Could you check a few things on this drawing? It's one solid part, dimensions in mm from its lowest x, y, z. A direction names the side the tool comes from. Give positions to 0.01 mm unless a question says otherwise; leave off trailing zeros. Loops run counter-clockwise (first coordinate to the right, second up) from the corner with the lowest first, then second, coordinate; pieces in that order, holes last. Notation, with made-up numbers: M -10,60.5 L 1,60.5 A20 cw 1,92.5 Z; hole C 6,-6 d4. An arc over 180 degrees is marked long. Answer as CSV lines item,"result". Start each with the question number.
Item 1: Will these pins go through, and if not, where does the flat tip stop? P1, Ø1, axis at x = 4.5, y = 6.5, coming from the +Z side; P2, Ø1, axis at x = 1, y = 4, coming from the +Z side; P3, Ø1.3, axis at x = 5, y = 4, coming from the +Z side; P4, Ø2, axis at x = 2.5, z = 4, coming from the +Y side (1 decimal).
Item 2: I want a section at A-A on z = 3.75. List the corners of the cut face in (x, y) for me (1 decimal).
Item 3: For the marked faces 1, 2 and 3, which set-ups out of +Z, -Z, +X, -X, +Y, -Y let a thin tool reach every point of the face, with its end or its side?
Item 4: I want a section at D-D on x = 1.5. List the corners of the cut face in (y, z) for me (1 decimal).
Item 5: I want a section at C-C on z = 1. List the corners of the cut face in (x, y) for me (1 decimal), plus the area to 3 significant figures.
Item 6: If I drill on line 1 along X through (y, z) = (5, 4.75); line 2 along Y through (x, z) = (4.5, 1.5) (1 decimal); line 3 along Z through (x, y) = (5.5, 3.25), over which ranges is the centre line in solid material (lowest first)? Write a range as from..to.
Item 7: I want a section at B-B on y = 1.5. List the corners of the cut face in (x, z) for me.
Item 8: If we mould it in two halves opening along X, with no side actions, what happens to the marked faces 4, 5 and 6? For each: released by +X, released by -X, zero draft, split by the parting line, or undercut.
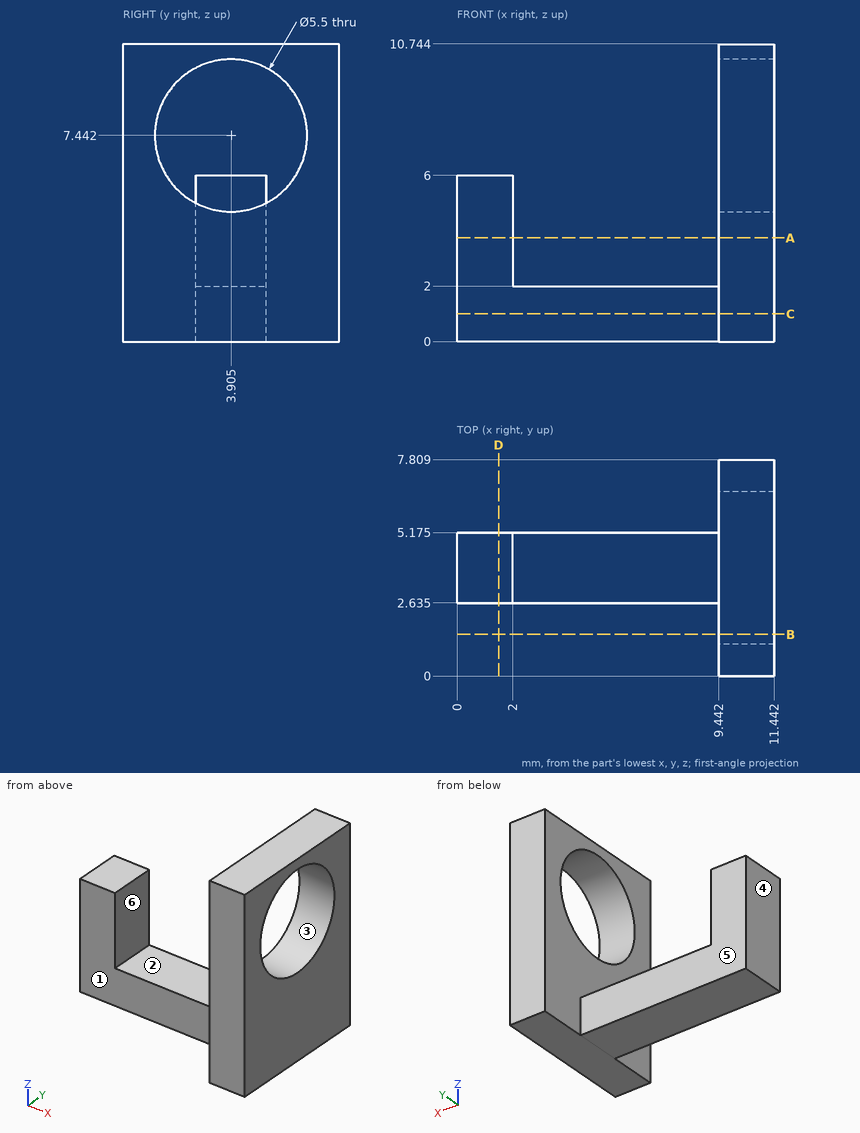
Result:
1,P1,"through"
1,P2,"z = 6"
1,P3,"z = 2"
1,P4,"y = 5.2"
2,outline,"M 0,2.6 L 2,2.6 L 2,5.2 L 0,5.2 Z; M 9.4,0 L 11.4,0 L 11.4,7.8 L 9.4,7.8 Z"
3,face 1,"+Z, -Z, -X, -Y"
3,face 2,"+Z, +Y, -Y"
3,face 3,"+X"
4,outline,"M 2.6,0 L 5.2,0 L 5.2,6 L 2.6,6 Z"
5,outline,"M 0,2.6 L 9.4,2.6 L 9.4,0 L 11.4,0 L 11.4,7.8 L 9.4,7.8 L 9.4,5.2 L 0,5.2 Z"
5,area,"39.6 mm^2"
6,line 1,"0..2, 9.44..11.44"
6,line 2,"2.6..5.2"
6,line 3,"0..2"
7,outline,"M 9.44,0 L 11.44,0 L 11.44,6.11 L 9.44,6.11 Z; M 9.44,8.78 L 11.44,8.78 L 11.44,10.74 L 9.44,10.74 Z"
8,face 4,"released by -X"
8,face 5,"zero draft"
8,face 6,"undercut"
